```python
from build123d import *

# Parameters (mm, degrees)
F0_W     = 44
F0_H     = 44
F0_W_2   = 39
F0_H_2   = 39
F1_DEPTH = 150
F3_D     = 8.8
F5_DEPTH = 19
F6_R     = 25
F8_D     = 52
F10_D    = 8.8


with BuildPart() as f1:
    # F0 (on Top) → F1 (new body)
    with BuildSketch(Plane.XY):
        Rectangle(F0_W, F0_H)
        Rectangle(F0_W_2, F0_H_2, mode=Mode.SUBTRACT)
    extrude(amount=F1_DEPTH)

    # F3 (through all)
    with Locations(Plane(origin=(-22, 0, 0), x_dir=(0, -1, 0), z_dir=(-1, 0, 0))):
        with Locations((0, 125), (0, 25)):
            Hole(F3_D / 2)

    # F4 (on Right) → F5 (join, symmetric)
    with BuildSketch(Plane.YZ):
        Polygon((-22, 12.5), (-22, 137.5), (-522, 137.5), (-522, 62.5), align=None)
    extrude(amount=F5_DEPTH, both=True)

    # F6
    f6_edges = [f1.edges().sort_by_distance(p)[0] for p in [
        (0, -522, 137.5),
        (0, -522, 62.5),
    ]]
    fillet(f6_edges, radius=F6_R)

    # F8 (through all)
    with Locations(Plane(origin=(-19, 0, 0), x_dir=(0, -1, 0), z_dir=(-1, 0, 0))):
        with Locations((484.5, 98.8123445264), (237, 98.8123445264)):
            Hole(F8_D / 2)

    # F10 (through all)
    with Locations(Plane.XY.offset(137.5)):
        with Locations((0, -237), (0, -484.5)):
            Hole(F10_D / 2)


solid = f1.part
```
The listing builds one solid part. Answer for the finished solid, in the listing's coordinates (mm). A direction names the side the tool comes from. Coordinates: 2 decimals unless noted, no trailing zeros. Loops run counter-clockwise (first coordinate to the right, second up) from the corner with the lowest first, then second, coordinate; pieces in that order, holes last. Notation, with made-up numbers: (30.25, 28) -> (86.25, 28) arc R28 ccw to (86.25, 65) -> close; hole circle Ø9 at (39, 23). An arc over 180 degrees is marked (long way). Return JSON: item names as keys, results as strings. Group by question number.
(1) Which of the six approach directions +Z, -Z, +X, -X, +Y, -Y give full straight-line access (tool end or side, diameter ignored) to faces 5 (the flat face through (-22, 0, 74)), 6 (the flat face through (0, -19.5, 74)), 7 (the flat face through (0, -256, 137.5)), 8 (the cylindrical face through (0.27, -490.14, 73.43)), 9 (the flat face through (-19, -220, 76))?
(2) Find the intervals of material crossed by probe 1 along Z at (x, y) = (21.25, 0); probe 2 along Y at (x, z) = (-0.5, 140.5); probe 3 along Y at (x, z) = (0, 62.5), in increasing order. Write a range as from..to.
(3) Given pin 1 Ø12 at (x, y) = (4, -338) entering from +Z; pin 2 Ø14 at (x, y) = (0, -237) entering from -Z; pin 3 Ø1 at (y, z) = (-45, 107) entering from +X, each flat-ended and moving along its own axis, determine where each tip first touches the part or whether it passes through.
(4) A cutting plane is placed at A-A on y = -290.5. Write down the section's boundary in (x, z).
(5) A cutting plane is placed at B-B on y = -105.5. Write down the section's boundary in (x, z).
(6) Determine the mould class of faces 1 (the cylindrical face through (-2.365, -480.79, 65.604)), 2 (the cylindrical face through (20.768, 2.365, 28.71)), 3 (the flat face through (19, -220, 76)), 4 (the cylindrical face through (0.573, -232.637, 53.056)) for opening direction X: released by +X, released by -X, zero draft, split by the parting line, or undercut.
The answers:
{
 "1": {"face 5": "+Z, -Z, -X, +Y, -Y", "face 6": "+Z, -Z", "face 7": "+Z, +X, -X, -Y", "face 8": "+X, -X", "face 9": "+Z, -Z, -X, -Y"},
 "2": {"probe 1": "z = 0..20.6, 29.4..120.6, 129.4..150", "probe 2": "y = -22..-19.5, 19.5..22", "probe 3": "y = -507.64..-488.9, -480.1..-241.4, -232.6..-19.5, 19.5..22"},
 "3": {"pin 1": "stops at z = 137.5", "pin 2": "stops at z = 33.3", "pin 3": "stops at x = 19"},
 "4": {"outline": "(-19, 39.35) -> (19, 39.35) -> (19, 137.5) -> (-19, 137.5) -> close"},
 "5": {"outline": "(-19, 20.85) -> (19, 20.85) -> (19, 137.5) -> (-19, 137.5) -> close"},
 "6": {"face 1": "undercut", "face 2": "zero draft", "face 3": "released by +X", "face 4": "undercut"}
}
